Autodesk Inventor part; units mm, degrees
ref_plane "YZ Plane" through (0, 0, 0) normal (1, 0, 0) x (0, 1, 0)
ref_plane "XZ Plane" through (0, 0, 0) normal (0, 1, 0) x (-1, 0, 0)
ref_plane "XY Plane" through (0, 0, 0) normal (0, 0, 1) x (1, 0, 0)
sketch "Эскиз1" plane through (0, 0, 0) normal (0, 0, 1) x (1, 0, 0)
  line L0 (117.5766, 0) -> (-136.0871, 0) construction
  line L1 (0, 117.7947) -> (0, -152.0118) construction
  line L2 (0, 0) -> (90, 0) construction
  line L3 (65.2, 57.2) -> (61.2, 57.2) construction
  line L4 (65.2, 57.2) -> (65.2, 52.2) construction
  line L5 (75, 65.5) -> (75, 87.5)
  line L6 (75, 87.5) -> (77, 87.5)
  arc A0 (90, 74.5) -> (77, 87.5) centre (77, 74.5) ccw
  line L7 (90, 74.5) -> (90, 0)
  circle A1 centre (65.2, 57.2) radius 2.1
  circle A2 centre (81.1924, 78.6924) radius 2.1
  line L8 (90, 63.5) -> (90, 65.5)
  line L9 (75, 65.5) -> (61.2, 65.5)
  line L10 (66.2, 29.1) -> (66.2, 36.5)
  line L11 (66.2, 24.1) -> (66.2, 0)
  line L12 (66.2, 29.1) -> (66.2, 24.1)
  line L13 (71, 62.5) -> (71, 45.5)
  line L14 (71, 45.5) -> (71, 56.5)
  line L15 (87, 56.5) -> (87, 45.5)
  line L16 (87, 45.5) -> (74.2, 45.5)
  line L17 (74.2, 45.5) -> (74.2, 56.5)
  line L18 (74.2, 56.5) -> (87, 56.5)
  line L19 (87, 56.5) -> (87, 45.5)
  line L20 (87, 45.5) -> (87, 40.5)
  line L21 (87, 40.5) -> (71, 40.5)
  line L22 (71, 40.5) -> (71, 45.5)
  line L23 (87, 40.5) -> (79, 40.5)
  arc A3 (66.2, 24.7) -> (82, 40.5) centre (66.2, 40.5) ccw
  arc A4 (66.2, 30.7) -> (76, 40.5) centre (65.5077, 41.1923) ccw
  line L24 (80.6, 45.5) -> (83.35, 45.5)
  line L25 (83.35, 45.5) -> (76.85, 45.5)
  line L26 (74.2, 45.5) -> (73.7, 45.5)
  circle A5 centre (76.85, 47) radius 0.5
  circle A6 centre (83.35, 47) radius 0.5
  line L27 (87, 45.5) -> (87, 55.9)
  line L28 (65.2, -57.2) -> (61.2, -57.2) construction
  line L29 (65.2, -57.2) -> (65.2, -52.2) construction
  line L30 (75, -65.5) -> (75, -87.5)
  line L31 (75, -87.5) -> (77, -87.5)
  arc A7 (77, -87.5) -> (90, -74.5) centre (77, -74.5) ccw
  line L32 (90, -74.5) -> (90, 0)
  circle A8 centre (65.2, -57.2) radius 2.1
  circle A9 centre (81.1924, -78.6924) radius 2.1
  line L33 (90, -63.5) -> (90, -65.5)
  line L34 (75, -65.5) -> (61.2, -65.5)
  line L35 (71, -62.5) -> (71, -45.5)
  line L36 (71, -45.5) -> (71, -56.5)
  line L37 (87, -56.5) -> (87, -45.5)
  line L38 (87, -45.5) -> (74.2, -45.5)
  line L39 (74.2, -45.5) -> (74.2, -56.5)
  line L40 (74.2, -56.5) -> (87, -56.5)
  line L41 (87, -56.5) -> (87, -45.5)
  line L42 (87, -45.5) -> (87, -40.5)
  line L43 (87, -40.5) -> (71, -40.5)
  line L44 (71, -40.5) -> (71, -45.5)
  line L45 (87, -40.5) -> (79, -40.5)
  arc A10 (82, -40.5) -> (66.2, -24.7) centre (66.2, -40.5) ccw
  arc A11 (76, -40.5) -> (66.2, -30.7) centre (65.5077, -41.1923) ccw
  line L46 (80.6, -45.5) -> (83.35, -45.5)
  line L47 (83.35, -45.5) -> (76.85, -45.5)
  line L48 (74.2, -45.5) -> (73.7, -45.5)
  circle A12 centre (76.85, -47) radius 0.5
  circle A13 centre (83.35, -47) radius 0.5
  line L49 (87, -45.5) -> (87, -55.9)
  line L50 (87, -56.5) -> (90, -56.5)
  circle A14 centre (87.508, -59.5) radius 1
  circle A15 centre (81.1924, 68.6924) radius 1.3
  circle A16 centre (81.1924, -68.6924) radius 1.3
  line L51 (61.2, 65.5) -> (61.2, 52.2)
  arc A17 (66.2, 47.2) -> (61.2, 52.2) centre (61.2, 47.2) ccw
  line L52 (66.2, 47.2) -> (66.2, 36.5)
  line L53 (66.2, -29.1) -> (66.2, -36.5)
  line L54 (66.2, -24.1) -> (66.2, 0)
  line L55 (66.2, -29.1) -> (66.2, -24.1)
  line L56 (61.2, -65.5) -> (61.2, -52.2)
  arc A18 (61.2, -52.2) -> (66.2, -47.2) centre (61.2, -47.2) ccw
  line L57 (66.2, -47.2) -> (66.2, -36.5)
  line L58 (85, -68.6924) -> (85, -84.747)
  line L59 (71, -62.5) -> (85, -62.5)
  line L60 (85, -62.5) -> (85, -68.6924)
  circle A19 centre (87.508, 59.5) radius 1
  line L61 (85, 68.6924) -> (85, 84.747)
  line L62 (71, 62.5) -> (85, 62.5)
  line L63 (85, 62.5) -> (85, 68.6924)
  line L64 (87, 56.5) -> (90, 56.5)
  point P0 (60.2, 65.5)
  point P1 (74.2, 55.9)
  point P2 (87, 82.8066)
  point P3 (60.2, -65.5)
  point P4 (74.2, -55.9)
  point P5 (87, -82.8066)
  point P6 (81.1924, 67.6924)
  point P7 (81.1924, -67.6924)
  point P8 (87.75, -59.5)
  dimension "d6" = 90
  dimension "d11" = 4
  dimension "d12" = 5
  dimension "d14" = 13
  dimension "d20" = 4.2
  dimension "d64" = 7.4
  dimension "d76" = 16
  dimension "d77" = 17
  dimension "d78" = 11
  dimension "d79" = 12.8
  dimension "d80" = 5
  dimension "d81" = 8
  dimension "d88" = 0.5
  dimension "d92" = 10.4
  dimension "d105" = 2.6
  dimension "d122" = 1
  dimension "d123" = 1
  dimension "d124" = 1
extrude "Выдавливание13" add sketch "Эскиз1" along normal blind 9 contours L5 L6 A0 L61 L63 L62 L13 L22 L21 A4 L10 L52 A17 L51 L9 | L7 L32 L50 L37 L42 L43 A10 L55 L54 L11 L12 A3 L21 L20 L15 L64 | A7 L31 L30 L34 L56 A18 L57 L53 A11 L43 L44 L35 L59 L60 L58 | A1 | A2 | A8 | A9
extrude "Выдавливание16" add sketch "Эскиз1" along normal blind 2 contours A0 L7 L64 L18 L17 L16 L20 L21 L22 L13 L62 L63 L61 | A4 L21 A3 L12 L10 | L15 L16 L17 L18 | L32 A7 L58 L60 L59 L35 L44 L43 L42 L38 L39 L40 L50 | L40 L39 L38 L37 | A10 L43 A11 L53 L55
fillet "Сопряжение3" radius 2 4 edges at (72.943, -33.757, 2) (77.3723, -29.3277, 2) (77.3723, 29.3277, 2) (72.943, 33.757, 2)
properties part number "front_part"
Model file for the job. Use its own axes, mm. A direction names the side the tool comes from. Round coordinates to 2 decimals unless told otherwise and drop trailing zeros. Order: outer loops, then holes, each group sorted by start corner. A loop starts at its lowest first (then second) coordinate and runs counter-clockwise, first axis right, second up. Notation, with made-up numbers: (88.5, 46.5) -> (97.5, 46.5) arc R14 ccw to (97.5, 73.5) -> close; hole circle Ø8 at (39, 17.5). An arc over 180 degrees is marked (long way). Use one line per item in the form item = value.
Item 1: Drill centre lines: line 1 (Y direction, x = 76.85, z = 1.65); line 2 (X direction, y = 47, z = 0.85); line 3 (X direction, y = 47, z = 6.5). Where is each one in solid material? Low to high.
Returned:
line_1 = -87.5 to -47.5, -46.5 to 46.5, 47.5 to 87.5
line_2 = 66.2 to 76.35, 77.35 to 82.85, 83.85 to 90
line_3 = 66.2 to 71, 87 to 90
Item 2: Cut at A-A, the plane z = 5.5. Give the number of separate pieces and of enclosed holes in the cut face, and give its area (3 significant figures).
Returned:
separate_pieces = 3
enclosed_holes = 2
area = 2,660 mm^2
Item 3: Flat gauge pins, fed straight in: pin 1 Ø4 at (x, z) = (81.5, 1) entering from -Y; pin 2 Ø5 at (x, z) = (85.5, 5) entering from +Y; pin 3 Ø3.5 at (x, z) = (84, 4) entering from -Y; pin 4 Ø12 at (x, y) = (79, 45) entering from +Z. Where does each tip first touch, or does it go through?
Returned:
pin_1 = -87.26
pin_2 = 86.03
pin_3 = -86.39
pin_4 = 9
Item 4: Pull direction Y, two halves, no side cores. Call faces 4 (the face through (87, -49, 5)), 5 (the face through (82.364, 86.342, 3.437)), 6 (the face through (77.494, 29.451, 6.465)), 7 (the face through (68, -65.5, 4)): released by +Y, released by -Y, zero draft, split by the parting line, or undercut.
Returned:
face_4 = zero draft
face_5 = released by +Y
face_6 = undercut
face_7 = released by -Y
Item 5: Cut at B-B, the plane y = -8.5. Write the cut outline in (x, z), and give its area (3 significant figures).
Returned:
outline = (66.2, 0) -> (90, 0) -> (90, 9) -> (66.2, 9) -> close
area = 214 mm^2
Item 6: Tool access for faces 1 (the face through (64.7, 50.77, 4.44)), 2 (the face through (84, -40.5, 5)), 3 (the face through (78, -62.5, 5)): list every direction of +Z, -Z, +X, -X, +Y, -Y with a clear straight run to the whole face (end or side of a thin tool).
Returned:
face_1 = +Z, -Z, -X
face_2 = +Z
face_3 = +Z, +X
